Check sheet for the drawn part. Datum: minimum x, y, z corner. Units: mm. A direction names the side the tool comes from. Give positions to 0.01 mm unless a question says otherwise; leave off trailing zeros. Loops run counter-clockwise (first coordinate to the right, second up) from the corner with the lowest first, then second, coordinate; pieces in that order, holes last. Notation, with made-up numbers: (31, 67) - (58, 67) arc R11 cw to (58, 71) - close; hole circle Ø9 at (28.5, -2). An arc over 180 degrees is marked (long way). Use one line per item in the form item = value.
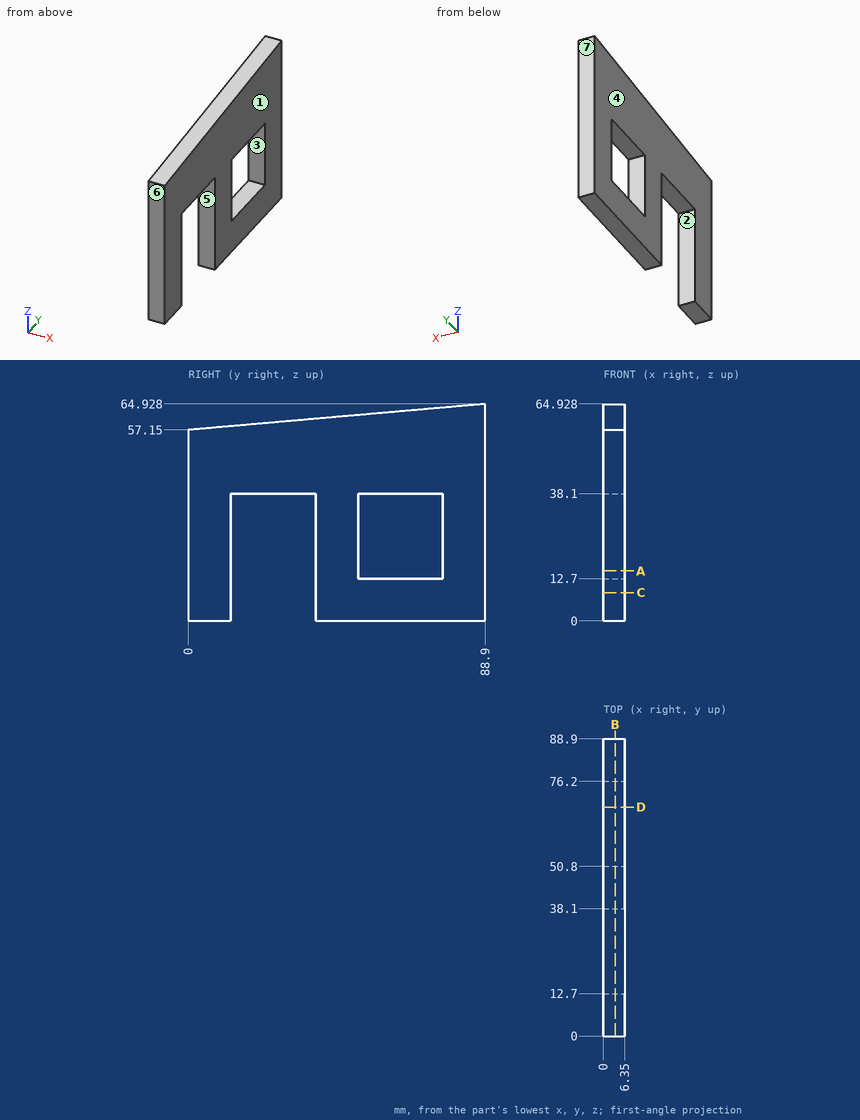
Item 1: Section check C-C on z = 8.5. Record the boundary of the cut face in (x, y), then the cut area to 3 significant figures.
Answer block:
outline = (0, 0) - (6.35, 0) - (6.35, 12.7) - (0, 12.7) - close; (0, 38.1) - (6.35, 38.1) - (6.35, 88.9) - (0, 88.9) - close
area = 403 mm2
Item 2: Access from +Z, -Z, +X, -X, +Y, -Y to the whole of each face (thin tool, end or side, straight path). Record for the marked faces 1, 2 and 3.
Answer block:
face_1 = +Z, -Z, +X, +Y, -Y
face_2 = -Z, +X, -X
face_3 = +X, -X
Item 3: Section check D-D on y = 68.5. Record the boundary of the cut face in (x, z).
Answer block:
outline = (0, 0) - (6.35, 0) - (6.35, 12.7) - (0, 12.7) - close; (0, 38.1) - (6.35, 38.1) - (6.35, 63.14) - (0, 63.14) - close
Item 4: Section check B-B on x = 3.5. Record the boundary of the cut face in (y, z), then the cut area to 3 significant figures.
Answer block:
outline = (0, 0) - (12.7, 0) - (12.7, 38.1) - (38.1, 38.1) - (38.1, 0) - (88.9, 0) - (88.9, 64.93) - (0, 57.15) - close; hole (50.8, 12.7) - (76.2, 12.7) - (76.2, 38.1) - (50.8, 38.1) - close
area = 3,810 mm2
Item 5: Thickness scan on L1, parallel to Y at x = 6.25, z = 13.5; L2, parallel to Y at x = 0.75, z = 12; L3, parallel to Z at x = 4.75, y = 8. Record the ranges inside material, lowest first.
Answer block:
L1 = 0 to 12.7, 38.1 to 50.8, 76.2 to 88.9
L2 = 0 to 12.7, 38.1 to 88.9
L3 = 0 to 57.85
Item 6: Section check A-A on z = 15. Record the boundary of the cut face in (x, y), then the cut area to 3 significant figures.
Answer block:
outline = (0, 0) - (6.35, 0) - (6.35, 12.7) - (0, 12.7) - close; (0, 38.1) - (6.35, 38.1) - (6.35, 50.8) - (0, 50.8) - close; (0, 76.2) - (6.35, 76.2) - (6.35, 88.9) - (0, 88.9) - close
area = 242 mm2
Item 7: Gauge pin test, flat ends, axial feed: P1, Ø1.9, axis at x = 2, y = 24.5, coming from the -Z side; P2, Ø3, axis at x = 4, y = 62.5, coming from the +Z side; P3, Ø8, axis at y = 30.5, z = 11, coming from the -X side. Record the tip position at first contact, or that the pin passes through.
Answer block:
P1 = 38.1
P2 = 62.75
P3 = through
Item 8: Mould release check, pull along Y, two halves, no side actions. Record for the marked faces 4, 5, 6 and 7: released by +Y, released by -Y, zero draft, split by the parting line, or undercut.
Answer block:
face_4 = zero draft
face_5 = undercut
face_6 = released by -Y
face_7 = released by +Y
